```python
from build123d import *

# Parameters (mm, degrees)
SKETCH1_W           = 110
SKETCH1_H           = 60
BOSS_EXTRUDE1_DEPTH = 2
SKETCH2_W           = 15
SKETCH2_H           = 13
BOSS_EXTRUDE2_DEPTH = 12
SKETCH3_W           = 6
SKETCH3_H           = 22.239539295
SKETCH3_H_2         = 21.340972051
BOSS_EXTRUDE3_DEPTH = 6
SKETCH4_W           = 7.81140843
SKETCH4_H           = 49.385459964
BOSS_EXTRUDE4_DEPTH = 10


with BuildPart() as part:
    # Sketch1 → Boss-Extrude1 (new body)
    with BuildSketch(Plane(origin=(0, 0, 0), x_dir=(1, 0, 0), z_dir=(0, 1, 0))):
        with Locations((3.029999611, 10.181542367)):
            Rectangle(SKETCH1_W, SKETCH1_H)
    extrude(amount=BOSS_EXTRUDE1_DEPTH)

    # Sketch2 → Boss-Extrude2 (add)
    with BuildSketch(Plane(origin=(0, 2, 0), x_dir=(1, 0, 0), z_dir=(0, 1, 0))):
        with Locations((50.529999611, 21.681542367)):
            Rectangle(SKETCH2_W, SKETCH2_H)
    extrude(amount=BOSS_EXTRUDE2_DEPTH)

    # Sketch3 → Boss-Extrude3 (add)
    with BuildSketch(Plane(origin=(0, 2, 0), x_dir=(1, 0, 0), z_dir=(0, 1, 0))):
        with Locations((28.757795867, 21.975237447)):
            Rectangle(SKETCH3_W, SKETCH3_H)
        with Locations((12.757795867, 21.975237447)):
            Rectangle(SKETCH3_W, SKETCH3_H)
        with Locations((-3.242204133, 21.975237447)):
            Rectangle(SKETCH3_W, SKETCH3_H)
        with Locations((-19.242204133, 21.975237447)):
            Rectangle(SKETCH3_W, SKETCH3_H)
        with Locations((48.599622808, -5.655705314)):
            Rectangle(SKETCH3_W, SKETCH3_H_2)
        with Locations((31.302203356, -5.655705314)):
            Rectangle(SKETCH3_W, SKETCH3_H_2)
        with Locations((12.757795867, -5.655705314)):
            Rectangle(SKETCH3_W, SKETCH3_H_2)
        with Locations((-3.242204133, -5.655705314)):
            Rectangle(SKETCH3_W, SKETCH3_H_2)
    extrude(amount=BOSS_EXTRUDE3_DEPTH)

    # Sketch4 → Boss-Extrude4 (add)
    with BuildSketch(Plane(origin=(0, 2, 0), x_dir=(1, 0, 0), z_dir=(0, 1, 0))):
        with Locations((-40.974267879, 8.402277113)):
            Rectangle(SKETCH4_W, SKETCH4_H)
    extrude(amount=BOSS_EXTRUDE4_DEPTH)


solid = part.part
```
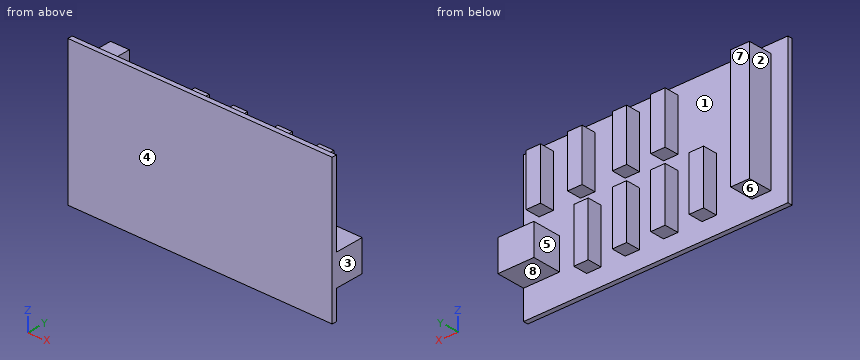
Can you work these out from the model? Positions are in its coordinate system, mm. Face numbers are marked on the shaded views. A direction names the side the tool comes from. Round coordinates to 2 decimals unless told otherwise and drop trailing zeros. Order: outer loops, then holes, each group sorted by start corner. A loop starts at its lowest first (then second) coordinate and runs counter-clockwise, first axis right, second up.
(1) We'd pull the mould along X, two halves only. Please class the marked faces 1, 2, 3 and 4: +X half, -X half, draft (parallel to the pull), parting line (faces both ways), or undercut.
Results are:
face 1: undercut
face 2: -X half
face 3: +X half
face 4: draft
(2) If I drill on L1, parallel to X at y = 5, z = -25.5; L2, parallel to Z at x = 14, y = 2.25 (3 decimals); L3, parallel to Y at x = -13, z = 15.5, over which ranges is the centre line in solid material (lowest first)?
Results are:
L1: x = -44.88 to -37.07, -22.24 to -16.24, -6.24 to -0.24, 9.76 to 15.76, 25.76 to 31.76, 43.03 to 58.03
L2: z = -33.095 to -10.855, -5.015 to 16.326
L3: y = 0 to 2
(3) If we section it at D-D (x = -34): Please give me the cut outline in (y, z).
Results are:
outline: (0, -40.18) - (2, -40.18) - (2, 19.82) - (0, 19.82) - close
(4) I'm going to push flat-ended pins straight in: pin 1 (6.5 mm diameter, centred on x = 11.5, y = 6, fed in from -Z) (3 decimals); pin 2 (6.5 mm diameter, centred on x = 13.5, y = 5.5, fed in from +Z); pin 3 (3 mm diameter, centred on x = -4.5, z = -27, fed in from +Y). Where does each tip first touch, or does it pass through?
Results are:
pin 1: stops at z = -33.095
pin 2: stops at z = 16.33
pin 3: stops at y = 8
(5) If we section it at C-C (y = 4): Count the separate pieces of the cut face and the enclosed holes in it, plus the area to 3 significant figures.
Results are:
separate pieces: 10
enclosed holes: 0
area: 1,630 mm2
(6) If we section it at A-A (y = 10.25): Please give me the cut outline in (x, z) (3 decimals), plus the area to 3 significant figures.
Results are:
outline: (-44.88, -33.095) - (-37.069, -33.095) - (-37.069, 16.29) - (-44.88, 16.29) - close; (43.03, -28.182) - (58.03, -28.182) - (58.03, -15.182) - (43.03, -15.182) - close
area: 581 mm2
(7) If we section it at B-B (z = -23): Please give me the cut outline in (x, y), plus the area to 3 significant figures.
Results are:
outline: (-51.97, 0) - (58.03, 0) - (58.03, 14) - (43.03, 14) - (43.03, 2) - (31.76, 2) - (31.76, 8) - (25.76, 8) - (25.76, 2) - (15.76, 2) - (15.76, 8) - (9.76, 8) - (9.76, 2) - (-0.24, 2) - (-0.24, 8) - (-6.24, 8) - (-6.24, 2) - (-16.24, 2) - (-16.24, 8) - (-22.24, 8) - (-22.24, 2) - (-37.07, 2) - (-37.07, 12) - (-44.88, 12) - (-44.88, 2) - (-51.97, 2) - close
area: 622 mm2
(8) On a 3-axis mill with a long thin cutter (end or side, diameter ignored), from which of +Z, -Z, +X, -X, +Y, -Y can I reach the whole of each face in a straight line? I mean the marked faces 5, 6, 7 and 8. Say none if no direction works.
Results are:
face 5: +Z, -Z, +Y
face 6: -Z, +X, -X, +Y
face 7: +Z, -Z, -X, +Y
face 8: -Z, +X, +Y
